from build123d import *

# Parameters (mm, degrees)
SKETCH_1_R          = 3.9
SKETCH_1_R_2        = 2.2
SKETCH_1_R_3        = 1
EXTRUDE_1_DEPTH     = 0.8
SKETCH_1_4_R        = 2.2
SKETCH_1_4_R_2      = 1
EXTRUDE_2_DEPTH     = 3.2
FILLET_1_R          = 0.2
SKETCH_2_R          = 1.15
CUT_EXTRUDE_1_DEPTH = 0.5
CUT_EXTRUDE_2_REACH = 8.813


with BuildPart() as part:
    # Sketch 1 → Extrude 1 (new body)
    with BuildSketch(Plane.XY):
        Circle(SKETCH_1_R)
        Circle(SKETCH_1_R_2, mode=Mode.SUBTRACT)
        Circle(SKETCH_1_R_2)
        Circle(SKETCH_1_R_3, mode=Mode.SUBTRACT)
    extrude(amount=-EXTRUDE_1_DEPTH)

    # Sketch 1_4 → Extrude 2 (add)
    with BuildSketch(Plane.XY):
        Circle(SKETCH_1_4_R)
        Circle(SKETCH_1_4_R_2, mode=Mode.SUBTRACT)
    extrude(amount=EXTRUDE_2_DEPTH)

    # Fillet 1
    fillet_1_edges = [part.edges().sort_by_distance(p)[0] for p in [
        (-2.2, 0, 3.2),
    ]]
    fillet(fillet_1_edges, radius=FILLET_1_R)

    # Sketch 2 → Cut-Extrude 1 (cut)
    with BuildSketch(Plane(origin=(0, 0, -0.8), x_dir=(-1, 0, 0), z_dir=(0, 0, -1))):
        Circle(SKETCH_2_R)
    extrude(amount=-CUT_EXTRUDE_1_DEPTH, mode=Mode.SUBTRACT)

    # Sketch 3 → Cut-Extrude 2 (cut, up to next)
    with BuildSketch(Plane(origin=(0, 0, -0.8), x_dir=(-1, 0, 0), z_dir=(0, 0, -1)), mode=Mode.PRIVATE) as cut_extrude_2_sk1:
        with BuildLine():
            ThreePointArc((-2.711088342, 0.7), (-2.8, 0), (-2.711088342, -0.7))
            Line((-2.711088342, -0.7), (-2.085665361, -0.7))
            ThreePointArc((-2.085665361, -0.7), (-2.2, 0), (-2.085665361, 0.7))
            Line((-2.085665361, 0.7), (-2.711088342, 0.7))
        make_face()
    cut_extrude_2_tool1 = extrude(cut_extrude_2_sk1.sketch, amount=-CUT_EXTRUDE_2_REACH, mode=Mode.PRIVATE) & part.part
    # Sketch 3 → Cut-Extrude 2 (cut, up to next)
    with BuildSketch(Plane(origin=(0, 0, -0.8), x_dir=(-1, 0, 0), z_dir=(0, 0, -1)), mode=Mode.PRIVATE) as cut_extrude_2_sk2:
        with BuildLine():
            Line((2.085665361, -0.7), (2.711088342, -0.7))
            ThreePointArc((2.711088342, -0.7), (2.77768315, -0.352812019), (2.8, 0))
            ThreePointArc((2.8, 0), (2.77768315, 0.352812019), (2.711088342, 0.7))
            Line((2.711088342, 0.7), (2.085665361, 0.7))
            ThreePointArc((2.085665361, 0.7), (2.1712282, 0.354637988), (2.2, 0))
            ThreePointArc((2.2, 0), (2.1712282, -0.354637988), (2.085665361, -0.7))
        make_face()
    cut_extrude_2_tool2 = extrude(cut_extrude_2_sk2.sketch, amount=-CUT_EXTRUDE_2_REACH, mode=Mode.PRIVATE) & part.part
    # Sketch 3 → Cut-Extrude 2 (cut, up to next)
    with BuildSketch(Plane(origin=(0, 0, -0.8), x_dir=(-1, 0, 0), z_dir=(0, 0, -1)), mode=Mode.PRIVATE) as cut_extrude_2_sk3:
        with BuildLine():
            ThreePointArc((-2.711088342, 0.7), (-2.8, 0), (-2.711088342, -0.7))
            Line((-2.711088342, -0.7), (-2.085665361, -0.7))
            ThreePointArc((-2.085665361, -0.7), (-2.2, 0), (-2.085665361, 0.7))
            Line((-2.085665361, 0.7), (-2.711088342, 0.7))
        make_face()
    cut_extrude_2_tool3 = extrude(cut_extrude_2_sk3.sketch, amount=-CUT_EXTRUDE_2_REACH, mode=Mode.PRIVATE) & part.part
    # Sketch 3 → Cut-Extrude 2 (cut, up to next)
    with BuildSketch(Plane(origin=(0, 0, -0.8), x_dir=(-1, 0, 0), z_dir=(0, 0, -1)), mode=Mode.PRIVATE) as cut_extrude_2_sk4:
        with BuildLine():
            Line((2.085665361, -0.7), (2.711088342, -0.7))
            ThreePointArc((2.711088342, -0.7), (2.77768315, -0.352812019), (2.8, 0))
            ThreePointArc((2.8, 0), (2.77768315, 0.352812019), (2.711088342, 0.7))
            Line((2.711088342, 0.7), (2.085665361, 0.7))
            ThreePointArc((2.085665361, 0.7), (2.1712282, 0.354637988), (2.2, 0))
            ThreePointArc((2.2, 0), (2.1712282, -0.354637988), (2.085665361, -0.7))
        make_face()
    cut_extrude_2_tool4 = extrude(cut_extrude_2_sk4.sketch, amount=-CUT_EXTRUDE_2_REACH, mode=Mode.PRIVATE) & part.part
    add(cut_extrude_2_tool1.solids().sort_by_distance((2.466051, 0, -0.8))[0], mode=Mode.SUBTRACT)
    add(cut_extrude_2_tool2.solids().sort_by_distance((-2.466051, 0, -0.8))[0], mode=Mode.SUBTRACT)
    add(cut_extrude_2_tool3.solids().sort_by_distance((2.466051, 0, -0.8))[0], mode=Mode.SUBTRACT)
    add(cut_extrude_2_tool4.solids().sort_by_distance((-2.466051, 0, -0.8))[0], mode=Mode.SUBTRACT)


solid = part.part
The model under review builds one solid part; all positions refer to its coordinate system, in mm. A direction names the side the tool comes from. Round coordinates to 2 decimals unless told otherwise and drop trailing zeros. Loops run counter-clockwise (first coordinate to the right, second up) from the corner with the lowest first, then second, coordinate; pieces in that order, holes last. Notation, with made-up numbers: (28, 26.25) -> (43, 26.25) arc R24 cw to (43, 52.25) -> close; hole circle Ø6 at (-22.5, -35.5). An arc over 180 degrees is marked (long way). One line per question, with ' | ' between items. Start each with the question number.
Item 1: Add section A-A, the plane x = 0. Write out the cut boundary in (y, z).
Item 2: Add section C-C, the plane z = 1. Write out the cut boundary in (x, y), then the cut area to 3 significant figures.
Item 3: Draft analysis for pull direction X (two halves, no side actions). For faces 3 (the face through (-2.87, 2.64, -0.39)), 4 (the face through (-1, -1, -0.8)), 5 (the face through (0, -1, 1)), 6 (the face through (0.91, -0.7, -0.55)), state which applies: +X half, -X half, draft (parallel to the pull), parting line (faces both ways), or undercut.
Item 4: Add section D-D, the plane x = 2.5. Write out the cut boundary in (y, z).
Item 5: For pin 1 (2.5 mm diameter, centred on x = 0, y = 0, fed in from -Z); pin 2 (1 mm diameter, centred on x = 2, z = 0, fed in from -Y); pin 3 (0.7 mm diameter, centred on x = 2.5, z = -0.5, fed in from +Y); pin 4 (1 mm diameter, centred on x = 2.5, z = 2, fed in from +Y), all flat-tipped, find the tip position at first contact; note any pin that passes through.
Item 6: Wall thickness on line 1 along Y through (x, z) = (0, 0.6); line 2 along Y through (x, z) = (0, -0.6): over which ranges is each line inside the solid? List them lowest first. Write a range as [from, to].
Item 7: Add section B-B, the plane z = -0.1. Write out the cut boundary in (x, y), then the cut area to 3 significant figures.
Item 8: Machinability: for faces 1 (the face through (2, -2, 0)), 2 (the face through (1, -1, 3.2)), which of the approach directions +Z, -Z, +X, -X, +Y, -Y give a long, thin tool a straight path to every point of the face, cutting with its end or side? Answer none if there is none.
Return value:
1) outline: (-3.9, -0.8) -> (-1.15, -0.8) -> (-1.15, -0.3) -> (-1, -0.3) -> (-1, 3.2) -> (-2, 3.2) arc R0.2 ccw to (-2.2, 3) -> (-2.2, 0) -> (-3.9, 0) -> close; (1, -0.3) -> (1.15, -0.3) -> (1.15, -0.8) -> (3.9, -0.8) -> (3.9, 0) -> (2.2, 0) -> (2.2, 3) arc R0.2 ccw to (2, 3.2) -> (1, 3.2) -> close
2) outline: circle Ø4.4 at (0, 0); hole circle Ø2 at (0, 0) | area: 12.1 mm2
3) face 3: parting line | face 4: draft | face 5: undercut | face 6: undercut
4) outline: (-2.99, -0.8) -> (-0.7, -0.8) -> (-0.7, 0) -> (-2.99, 0) -> close; (0.7, -0.8) -> (2.99, -0.8) -> (2.99, 0) -> (0.7, 0) -> close
5) pin 1: stops at z = -0.8 | pin 2: stops at y = -3.6 | pin 3: stops at y = 3.25 | pin 4: stops at y = 0.92
6) line 1: y = [-2.2, -1], [1, 2.2] | line 2: y = [-3.9, -1.15], [1.15, 3.9]
7) outline: circle Ø7.8 at (0, 0); hole (-2.71, -0.7) -> (-2.09, -0.7) arc R2.2 cw to (-2.09, 0.7) -> (-2.71, 0.7) arc R2.8 ccw to start; hole circle Ø2 at (0, 0); hole (2.09, -0.7) -> (2.71, -0.7) arc R2.8 ccw to (2.71, 0.7) -> (2.09, 0.7) arc R2.2 cw to start | area: 42.9 mm2
8) face 1: +Z | face 2: +Z, +X, -X, +Y, -Y
